For this review, take the finished solid that the model builds, in its own axes (mm). Give positions to 0.01 mm unless a question says otherwise; leave off trailing zeros. Order: outer loops, then holes, each group sorted by start corner. A loop starts at its lowest first (then second) coordinate and runs counter-clockwise, first axis right, second up. Notation, with made-up numbers: (71.5, -10) -> (83.5, -10) arc R23 ccw to (83.5, 21) -> close; hole circle Ø9 at (25.5, 10.5). An arc over 180 degrees is marked (long way). Use CSV: the item, a comma, the result in double quotes. Start each with the question number.
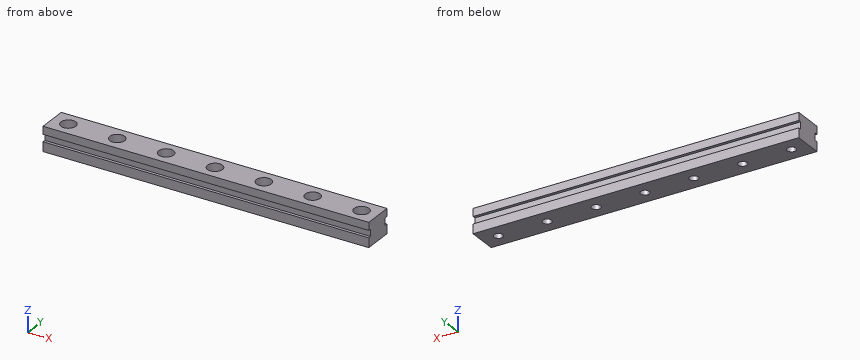
```python
from build123d import *

# Parameters (mm, degrees)
F_100_START                            = 27.5
F_100_MM_RAIL_BLANK_PROFILE_W          = 100
F_100_MM_RAIL_BLANK_PROFILE_H          = 9
F_100_MM_RAIL_BLANK_DEPTH              = 7.5
LONGITUDINAL_START                     = 30.4
LONGITUDINAL_RUNNING_GROOVES_PROFILE_W = 100.2
LONGITUDINAL_RUNNING_GROOVES_PROFILE_H = 1.4
LONGITUDINAL_RUNNING_GROOVES_DEPTH     = 2.2
RAIL_START                             = 27.4
RAIL_BOLT_CLEARANCE_PROFILE_R          = 1.35
RAIL_BOLT_CLEARANCE_DEPTH              = 7.8
RAIL_START_2                           = 32
RAIL_HEAD_RECESSES_PROFILE_R           = 2.3
RAIL_HEAD_RECESSES_DEPTH               = 3.2


with BuildPart() as part:
    # 100 mm rail blank profile → 100 mm rail blank (new body)
    with BuildSketch(Plane.XY.offset(F_100_START)):
        with Locations((33, 18.5)):
            Rectangle(F_100_MM_RAIL_BLANK_PROFILE_W, F_100_MM_RAIL_BLANK_PROFILE_H)
    extrude(amount=F_100_MM_RAIL_BLANK_DEPTH)

    # Longitudinal running grooves profile → Longitudinal running grooves (cut)
    with BuildSketch(Plane.XY.offset(LONGITUDINAL_START)):
        with Locations((33, 14.2)):
            Rectangle(LONGITUDINAL_RUNNING_GROOVES_PROFILE_W, LONGITUDINAL_RUNNING_GROOVES_PROFILE_H)
        with Locations((33, 22.8)):
            Rectangle(LONGITUDINAL_RUNNING_GROOVES_PROFILE_W, LONGITUDINAL_RUNNING_GROOVES_PROFILE_H)
    extrude(amount=LONGITUDINAL_RUNNING_GROOVES_DEPTH, mode=Mode.SUBTRACT)

    # Rail bolt clearance profile → Rail bolt clearance (cut)
    with BuildSketch(Plane.XY.offset(RAIL_START)):
        with Locations((-12, 18.5)):
            Circle(RAIL_BOLT_CLEARANCE_PROFILE_R)
        with Locations((3, 18.5)):
            Circle(RAIL_BOLT_CLEARANCE_PROFILE_R)
        with Locations((18, 18.5)):
            Circle(RAIL_BOLT_CLEARANCE_PROFILE_R)
        with Locations((33, 18.5)):
            Circle(RAIL_BOLT_CLEARANCE_PROFILE_R)
        with Locations((48, 18.5)):
            Circle(RAIL_BOLT_CLEARANCE_PROFILE_R)
        with Locations((63, 18.5)):
            Circle(RAIL_BOLT_CLEARANCE_PROFILE_R)
        with Locations((78, 18.5)):
            Circle(RAIL_BOLT_CLEARANCE_PROFILE_R)
    extrude(amount=RAIL_BOLT_CLEARANCE_DEPTH, mode=Mode.SUBTRACT)

    # Rail head recesses profile → Rail head recesses (cut)
    with BuildSketch(Plane.XY.offset(RAIL_START_2)):
        with Locations((-12, 18.5)):
            Circle(RAIL_HEAD_RECESSES_PROFILE_R)
        with Locations((3, 18.5)):
            Circle(RAIL_HEAD_RECESSES_PROFILE_R)
        with Locations((18, 18.5)):
            Circle(RAIL_HEAD_RECESSES_PROFILE_R)
        with Locations((33, 18.5)):
            Circle(RAIL_HEAD_RECESSES_PROFILE_R)
        with Locations((48, 18.5)):
            Circle(RAIL_HEAD_RECESSES_PROFILE_R)
        with Locations((63, 18.5)):
            Circle(RAIL_HEAD_RECESSES_PROFILE_R)
        with Locations((78, 18.5)):
            Circle(RAIL_HEAD_RECESSES_PROFILE_R)
    extrude(amount=RAIL_HEAD_RECESSES_DEPTH, mode=Mode.SUBTRACT)


solid = part.part
```
1. Clearance check with flat-ended pins moving along their axes: P1, Ø2, axis at x = 48, y = 18.5, coming from the -Z side; P2, Ø3.5, axis at x = 33, y = 18.5, coming from the +Z side; P3, Ø0.7, axis at x = 24.5, z = 31, coming from the -Y side. State where each tip first meets the part, or that it passes through.
2. Consider section B-B (z = 29.5). State the section outline as (x, y) points, plus the area to 3 significant figures.
3. Consider section D-D (y = 18.5). State how many separate pieces and enclosed holes the cut face has, plus the area to 3 significant figures.
4. Consider section A-A (x = 63). State the section outline as (y, z) points.
5. Consider section C-C (x = 23.5). State the section outline as (y, z) points.
6. To check wall thickness, follow L1, parallel to Y at x = 78, z = 34; L2, parallel to Z at x = -13, y = 14.75; L3, parallel to Y at x = 63, z = 30.8. State the ranges of each line that lie inside material, in increasing order. Write a range as [from, to].
Answer list:
1,P1,"through"
1,P2,"z = 32"
1,P3,"y = 14.9"
2,outline,"(-17, 14) -> (83, 14) -> (83, 23) -> (-17, 23) -> close; hole circle Ø2.7 at (-12, 18.5); hole circle Ø2.7 at (3, 18.5); hole circle Ø2.7 at (18, 18.5); hole circle Ø2.7 at (33, 18.5); hole circle Ø2.7 at (48, 18.5); hole circle Ø2.7 at (63, 18.5); hole circle Ø2.7 at (78, 18.5)"
2,area,"860 mm2"
3,separate pieces,"8"
3,enclosed holes,"0"
3,area,"568 mm2"
4,outline,"(14, 27.5) -> (17.15, 27.5) -> (17.15, 32) -> (16.2, 32) -> (16.2, 35) -> (14, 35) -> (14, 32.6) -> (14.9, 32.6) -> (14.9, 30.4) -> (14, 30.4) -> close; (19.85, 27.5) -> (23, 27.5) -> (23, 30.4) -> (22.1, 30.4) -> (22.1, 32.6) -> (23, 32.6) -> (23, 35) -> (20.8, 35) -> (20.8, 32) -> (19.85, 32) -> close"
5,outline,"(14, 27.5) -> (23, 27.5) -> (23, 30.4) -> (22.1, 30.4) -> (22.1, 32.6) -> (23, 32.6) -> (23, 35) -> (14, 35) -> (14, 32.6) -> (14.9, 32.6) -> (14.9, 30.4) -> (14, 30.4) -> close"
6,L1,"[14, 16.2], [20.8, 23]"
6,L2,"[27.5, 30.4], [32.6, 35]"
6,L3,"[14.9, 17.15], [19.85, 22.1]"
